from build123d import *

# Parameters (mm, degrees)
BASE_EXTRUDE_DEPTH    = 8
SKETCH4_R             = 3.4
M8_GEVINDHULLER_DEPTH = 10


with BuildPart() as part:
    # Sketch1 → Base-Extrude (new body)
    with BuildSketch(Plane.XY):
        with BuildLine():
            Line((17.5, -17.5), (17.5, -37.5))
            ThreePointArc((17.5, -37.5), (18.964466094, -41.035533906), (22.5, -42.5))
            Line((22.5, -42.5), (33, -42.5))
            ThreePointArc((33, -42.5), (36.535533906, -41.035533906), (38, -37.5))
            Line((38, -37.5), (38, -12.619678905))
            ThreePointArc((38, -12.619678905), (37.772116295, -10.01495624), (37.095389312, -7.489376755))
            Line((37.095389312, -7.489376755), (33.987127064, 1.050503583))
            ThreePointArc((33.987127064, 1.050503583), (24.834222454, 12.978801107), (10.494811545, 17.5))
            Line((10.494811545, 17.5), (-10.494811545, 17.5))
            ThreePointArc((-10.494811545, 17.5), (-24.834222454, 12.978801107), (-33.987127064, 1.050503583))
            Line((-33.987127064, 1.050503583), (-37.095389312, -7.489376755))
            ThreePointArc((-37.095389312, -7.489376755), (-37.772116295, -10.01495624), (-38, -12.619678905))
            Line((-38, -12.619678905), (-38, -37.5))
            ThreePointArc((-38, -37.5), (-36.535533906, -41.035533906), (-33, -42.5))
            Line((-33, -42.5), (-22.5, -42.5))
            ThreePointArc((-22.5, -42.5), (-18.964466094, -41.035533906), (-17.5, -37.5))
            Line((-17.5, -37.5), (-17.5, -17.5))
            ThreePointArc((-17.5, -17.5), (0, 0), (17.5, -17.5))
        make_face()
    extrude(amount=BASE_EXTRUDE_DEPTH)

    # Sketch4 → M8 gevindhuller (cut)
    with BuildSketch(Plane.XY.offset(8)):
        with Locations((-28, -14.5)):
            Circle(SKETCH4_R)
        with Locations((28, -14.5)):
            Circle(SKETCH4_R)
    extrude(amount=-M8_GEVINDHULLER_DEPTH, mode=Mode.SUBTRACT)


solid = part.part
Read the model definition and answer for the solid it produces. Units are mm, in the model's axes. A direction names the side the tool comes from. Give positions to 0.01 mm unless a question says otherwise; leave off trailing zeros. Write each loop counter-clockwise with the first axis right and the second up, starting at its lowest first coordinate (ties: lowest second). Pieces come first, ordered by that corner, then holes. Notation, with made-up numbers: (70, 6.5) - (84, 6.5) arc R21 cw to (84, 40.5) - close; hole circle Ø7 at (46, -22.75). An arc over 180 degrees is marked (long way). Answer in a Markdown table with one row per item. Add a question column.
Item 1: Determine the mould class of faces 3 (the face through (-38, -25, 4)), 4 (the face through (-26.4, -17.5, 4.1)), 5 (the face through (38, -25, 4)), 6 (the face through (18.93, -41, 3.94)) for opening direction X: pulls with the +X half, pulls with the -X half, needs draft (parallel to the pull), parting line crosses it, or undercut.
Item 2: Section B-B, the plane x = -28 is taken. Write down the section's boundary in (y, z), and give its area (3 significant figures).
Item 3: Find the intervals of material crossed by L1, parallel to X at y = -37, z = 1; L2, parallel to X at y = -10, z = 7.25; L3, parallel to X at y = -17, z = 5.5, in increasing order.
Item 4: Section D-D, the plane y = -14.5 is taken. Write down the section's boundary in (x, z), and give its area (3 significant figures).
Item 5: A tool of negligible diameter and unlimited length cuts with its end or side. For faces 1 (the face through (29.6, -17.5, 4.1)), 2 (the face through (-17.5, -28, 4)), from which of +Z, -Z, +X, -X, +Y, -Y can it reach the whole face along a straight path? Write none if from no direction.
Item 6: Section A-A, the plane y = -22 is taken. Write down the section's boundary in (x, z), and give its area (3 significant figures).
Item 7: Section C-C, the plane z = 6.75 is taken. Write down the section's boundary in (x, y), and give its area (3 significant figures).
Recorded:
| question | item | result |
|---|---|---|
| 1 | face 3 | pulls with the -X half |
| 1 | face 4 | undercut |
| 1 | face 5 | pulls with the +X half |
| 1 | face 6 | undercut |
| 2 | outline | (-42.5, 0) - (-17.9, 0) - (-17.9, 8) - (-42.5, 8) - close; (-11.1, 0) - (10.35, 0) - (10.35, 8) - (-11.1, 8) - close |
| 2 | area | 368 mm2 |
| 3 | L1 | x = -38 to -17.5, 17.5 to 38 |
| 3 | L2 | x = -37.77 to -15.81, 15.81 to 37.77 |
| 3 | L3 | x = -38 to -30.3, -25.7 to -17.49, 17.49 to 25.7, 30.3 to 38 |
| 4 | outline | (-38, 0) - (-31.4, 0) - (-31.4, 8) - (-38, 8) - close; (-24.6, 0) - (-17.24, 0) - (-17.24, 8) - (-24.6, 8) - close; (17.24, 0) - (24.6, 0) - (24.6, 8) - (17.24, 8) - close; (31.4, 0) - (38, 0) - (38, 8) - (31.4, 8) - close |
| 4 | area | 223 mm2 |
| 5 | face 1 | +Z, -Z |
| 5 | face 2 | +Z, -Z, -Y |
| 6 | outline | (-38, 0) - (-17.5, 0) - (-17.5, 8) - (-38, 8) - close; (17.5, 0) - (38, 0) - (38, 8) - (17.5, 8) - close |
| 6 | area | 328 mm2 |
| 7 | outline | (-38, -37.5) arc R5 ccw to (-33, -42.5) - (-22.5, -42.5) arc R5 ccw to (-17.5, -37.5) - (-17.5, -17.5) arc R17.5 cw to (17.5, -17.5) - (17.5, -37.5) arc R5 ccw to (22.5, -42.5) - (33, -42.5) arc R5 ccw to (38, -37.5) - (38, -12.62) arc R15 ccw to (37.1, -7.49) - (33.99, 1.05) arc R25 ccw to (10.49, 17.5) - (-10.49, 17.5) arc R25 ccw to (-33.99, 1.05) - (-37.1, -7.49) arc R15 ccw to (-38, -12.62) - close; hole circle Ø6.8 at (-28, -14.5); hole circle Ø6.8 at (28, -14.5) |
| 7 | area | 2,720 mm2 |
